from build123d import *

# Parameters (mm, degrees)
SKETCH_R     = 1.6
PAD_DEPTH    = 2.8
SKETCH001_R  = 1.25
HOLE_DEPTH   = 2.801
POCKET_DEPTH = 2.801


with BuildPart() as part:
    # Sketch → Pad (new body)
    with BuildSketch(Plane.XY):
        with BuildLine():
            Line((1, 0), (8, 0))
            Line((8, 0), (8, -2.3))
            ThreePointArc((8, -2.3), (8.146447, -2.653553), (8.5, -2.8))
            Line((8.5, -2.8), (18.1, -2.8))
            ThreePointArc((18.1, -2.8), (18.453553, -2.653553), (18.6, -2.3))
            Line((18.6, -2.3), (18.6, 0))
            Line((18.6, 0), (56.2, 0))
            Line((56.2, 0), (56.2, -2.3))
            ThreePointArc((56.2, -2.3), (56.346447, -2.653553), (56.7, -2.8))
            Line((56.7, -2.8), (66.3, -2.8))
            ThreePointArc((66.3, -2.8), (66.653553, -2.653553), (66.8, -2.3))
            Line((66.8, -2.3), (66.8, 0))
            Line((66.8, 0), (70.1, 0))
            ThreePointArc((70.1, 0), (70.453553, 0.146447), (70.6, 0.5))
            Line((70.6, 0.5), (70.6, 4.292893))
            ThreePointArc((70.746447, 4.646447), (70.63806, 4.484235), (70.6, 4.292893))
            Line((70.746447, 4.646447), (73.6, 7.5))
            Line((73.6, 7.5), (73.6, 34))
            Line((73.6, 34), (66.8, 40.8))
            Line((66.8, 40.8), (66.8, 65))
            ThreePointArc((66.8, 65), (66.653553, 65.353553), (66.3, 65.5))
            Line((66.3, 65.5), (63.5, 65.5))
            ThreePointArc((63.5, 65.5), (63.146447, 65.353553), (63, 65))
            Line((63, 65), (63, 62.7))
            Line((63, 62.7), (-1.2, 62.7))
            Line((-1.2, 62.7), (-1.2, 65))
            ThreePointArc((-1.2, 65), (-1.346447, 65.353553), (-1.7, 65.5))
            Line((-1.7, 65.5), (-7.6, 65.5))
            ThreePointArc((-7.6, 65.5), (-7.953553, 65.353553), (-8.1, 65))
            Line((-8.1, 65), (-8.1, 46.9))
            ThreePointArc((-8.1, 46.9), (-7.807107, 46.192893), (-7.1, 45.9))
            Line((-7.1, 45.9), (6.7, 45.9))
            ThreePointArc((7.7, 44.9), (7.407107, 45.607107), (6.7, 45.9))
            Line((7.7, 44.9), (7.7, 31))
            ThreePointArc((6.7, 30), (7.407107, 30.292893), (7.7, 31))
            Line((6.7, 30), (-7.1, 30))
            ThreePointArc((-7.1, 30), (-7.807107, 29.707107), (-8.1, 29))
            Line((-8.1, 29), (-8.1, 1))
            ThreePointArc((-8.1, 1), (-7.807107, 0.292893), (-7.1, 0))
            Line((-7.1, 0), (1, 0))
        make_face()
        with Locations((5.1, 57.9)):
            Circle(SKETCH_R, mode=Mode.SUBTRACT)
        with Locations((63.1, 57.9)):
            Circle(SKETCH_R, mode=Mode.SUBTRACT)
        with Locations((5.1, 8.9)):
            Circle(SKETCH_R, mode=Mode.SUBTRACT)
        with Locations((63.1, 8.9)):
            Circle(SKETCH_R, mode=Mode.SUBTRACT)
    extrude(amount=PAD_DEPTH)

    # Sketch001 (on Face46 of Pad) → Hole (cut, through all)
    with BuildSketch(Plane.XY.offset(2.8)):
        with Locations((12.3, 57.9)):
            Circle(SKETCH001_R)
        with Locations((12.3, 34.3)):
            Circle(SKETCH001_R)
        with Locations((63.1, 34.3)):
            Circle(SKETCH001_R)
        with Locations((63.1, 57.9)):
            Circle(SKETCH001_R)
        with Locations((13, 26.2)):
            Circle(SKETCH001_R)
        with Locations((13, 7.2)):
            Circle(SKETCH001_R)
        with Locations((69, 7.2)):
            Circle(SKETCH001_R)
        with Locations((69, 26.2)):
            Circle(SKETCH001_R)
    extrude(amount=-HOLE_DEPTH, mode=Mode.SUBTRACT)

    # Sketch002 (on Face5 of Hole) → Pocket (cut, through all)
    with BuildSketch(Plane.XY.offset(2.8)):
        with BuildLine():
            Line((57.1, 56.7), (19, 56.7))
            ThreePointArc((19, 56.7), (17.585786, 56.114214), (17, 54.7))
            Line((17, 54.7), (17, 26.2))
            ThreePointArc((13, 22.2), (15.828427, 23.371573), (17, 26.2))
            Line((-2.1, 22.2), (13, 22.2))
            Line((-2.1, 12), (-2.1, 22.2))
            Line((13, 12), (-2.1, 12))
            ThreePointArc((17.8, 7.2), (16.394113, 10.594113), (13, 12))
            Line((17.8, 7.2), (17.8, 6))
            Line((17.8, 6), (59.1, 6))
            Line((59.1, 6), (59.1, 9.4))
            ThreePointArc((62.6, 12.9), (60.125126, 11.874874), (59.1, 9.4))
            Line((63, 12.9), (62.6, 12.9))
            ThreePointArc((63, 12.9), (64.414214, 13.485786), (65, 14.9))
            Line((65, 28.3), (65, 14.9))
            ThreePointArc((65, 28.3), (64.414214, 29.714214), (63, 30.3))
            Line((62.6, 30.3), (63, 30.3))
            ThreePointArc((59.1, 33.8), (60.125126, 31.325126), (62.6, 30.3))
            Line((59.1, 33.8), (59.1, 54.7))
            ThreePointArc((59.1, 54.7), (58.514214, 56.114214), (57.1, 56.7))
        make_face()
    extrude(amount=-POCKET_DEPTH, mode=Mode.SUBTRACT)


solid = part.part
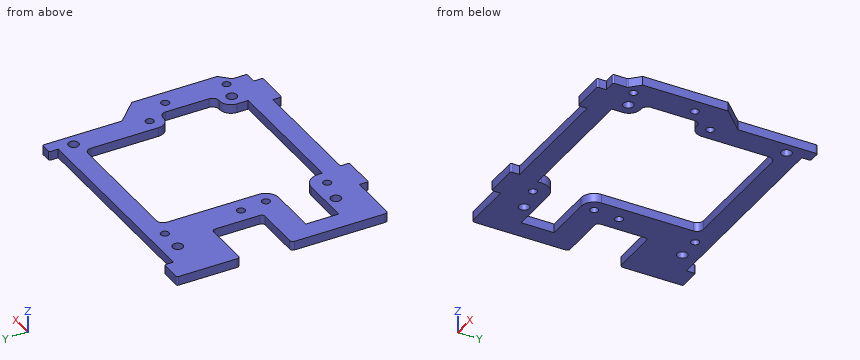
Design review of the part built by this model. Coordinates are the model's own, in mm. Round coordinates to 2 decimals unless told otherwise and drop trailing zeros. Write each loop counter-clockwise with the first axis right and the second up, starting at its lowest first coordinate (ties: lowest second). Pieces come first, ordered by that corner, then holes. Notation, with made-up numbers: M -15.75,68 L 32.25,68 A25 cw 32.25,102 Z; hole C -7,39.5 d8. An arc over 180 degrees is marked long. One line per item, written item: value. Start each with the question number.
1. Take a section at B-B on x = 5.1. State the section outline as (y, z) points.
2. Take a section at A-A on y = 19.5. State the section outline as (x, z) points.
3. Take a section at D-D on x = 46. State the section outline as (y, z) points.
4. Clearance check with flat-ended pins moving along their axes: P1, Ø0.8, axis at y = 3, z = 1, coming from the +X side; P2, Ø0.8, axis at x = 24.5, z = 1.5, coming from the +Y side; P3, Ø0.8, axis at x = 69, z = 2, coming from the -Y side; P4, Ø1.5, axis at x = 13, y = 7.2, coming from the -Z side. State where each tip first meets the part, or that it passes through.
5. To check wall thickness, follow probe 1 along X at (y, z) = (58, 2.05); probe 2 along Y at (x, z) = (14, 0.45); probe 3 along Y at (x, z) = (63.1, 1.2). State the ranges of each line that lie inside material, in increasing order. Write a range as from..to.
6. Take a section at C-C on y = 57.9. State the section outline as (x, z) points.
Computed:
1. outline: M 0,0 L 7.3,0 L 7.3,2.8 L 0,2.8 Z; M 10.5,0 L 12,0 L 12,2.8 L 10.5,2.8 Z; M 22.2,0 L 30,0 L 30,2.8 L 22.2,2.8 Z; M 45.9,0 L 56.3,0 L 56.3,2.8 L 45.9,2.8 Z; M 59.5,0 L 62.7,0 L 62.7,2.8 L 59.5,2.8 Z
2. outline: M -8.1,0 L -2.1,0 L -2.1,2.8 L -8.1,2.8 Z; M 65,0 L 73.6,0 L 73.6,2.8 L 65,2.8 Z
3. outline: M 0,0 L 6,0 L 6,2.8 L 0,2.8 Z; M 56.7,0 L 62.7,0 L 62.7,2.8 L 56.7,2.8 Z
4. P1: stops at x = 70.6
4. P2: stops at y = 62.7
4. P3: stops at y = 0
4. P4: passes through
5. probe 1: x = -8.1..3.5, 6.7..11.05, 13.55..61.5, 64.7..66.8
5. probe 2: y = -2.8..6.45, 7.95..11.89, 22.33..25.45, 26.95..62.7
5. probe 3: y = -2.8..7.3, 10.5..12.9, 30.3..33.05, 35.55..56.3, 59.5..65.3
6. outline: M -8.1,0 L 3.5,0 L 3.5,2.8 L -8.1,2.8 Z; M 6.7,0 L 11.05,0 L 11.05,2.8 L 6.7,2.8 Z; M 13.55,0 L 61.5,0 L 61.5,2.8 L 13.55,2.8 Z; M 64.7,0 L 66.8,0 L 66.8,2.8 L 64.7,2.8 Z
